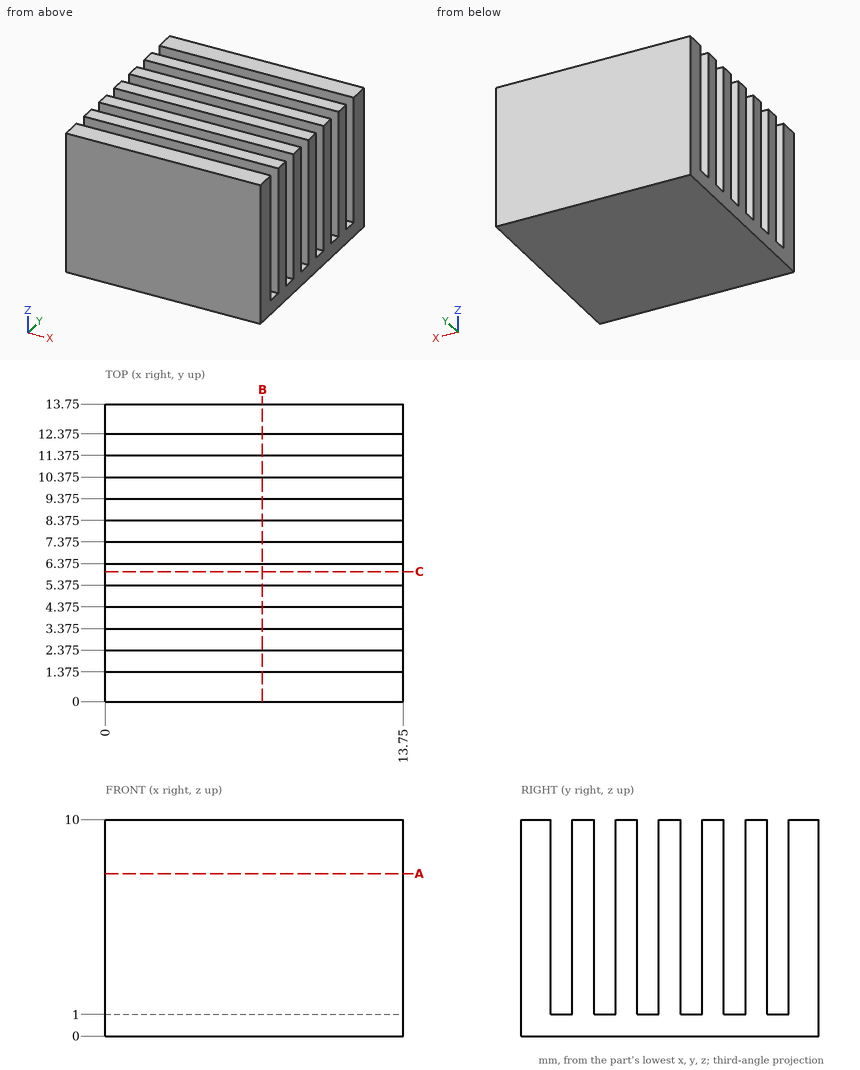
Geometry check sheet. Reference: drawing and pictorial views, mm from the part's lowest x, y, z. Round coordinates to 2 decimals unless told otherwise and drop trailing zeros. Loops run counter-clockwise (first coordinate to the right, second up) from the corner with the lowest first, then second, coordinate; pieces in that order, holes last. Notation, with made-up numbers: (87, 16.25) - (122, 16.25) arc R20 ccw to (122, 27.25) - close; hole circle Ø10 at (37, -5). An arc over 180 degrees is marked (long way). Answer in a Markdown table with one row per item. Add a question column.
Q1. Gauge pin test, flat ends, axial feed: pin 1 (1.1 mm diameter, centred on x = 9.5, y = 10, fed in from +Z); pin 2 (0.5 mm diameter, centred on x = 10, y = 6, fed in from +Z). Record the tip position at first contact, or that the pin passes through.
Q2. Section check A-A on z = 7.5. Enter the section's corners in (x, y) (3 decimals).
Q3. Section check B-B on x = 7.25. Enter the section's corners in (y, z) (3 decimals), plus the area to 3 significant figures.
Q4. Section check C-C on y = 6. Enter the section's corners in (x, z), plus the area to 4 significant figures.
Q5. Material ranges on line 1 (Z direction, x = 3, y = 7.5), recorded low to high.
Found:
| question | item | result |
|---|---|---|
| 1 | pin 1 | stops at z = 10 |
| 1 | pin 2 | stops at z = 1 |
| 2 | outline | (0, 0) - (13.75, 0) - (13.75, 1.375) - (0, 1.375) - close; (0, 2.375) - (13.75, 2.375) - (13.75, 3.375) - (0, 3.375) - close; (0, 4.375) - (13.75, 4.375) - (13.75, 5.375) - (0, 5.375) - close; (0, 6.375) - (13.75, 6.375) - (13.75, 7.375) - (0, 7.375) - close; (0, 8.375) - (13.75, 8.375) - (13.75, 9.375) - (0, 9.375) - close; (0, 10.375) - (13.75, 10.375) - (13.75, 11.375) - (0, 11.375) - close; (0, 12.375) - (13.75, 12.375) - (13.75, 13.75) - (0, 13.75) - close |
| 3 | outline | (0, 0) - (13.75, 0) - (13.75, 10) - (12.375, 10) - (12.375, 1) - (11.375, 1) - (11.375, 10) - (10.375, 10) - (10.375, 1) - (9.375, 1) - (9.375, 10) - (8.375, 10) - (8.375, 1) - (7.375, 1) - (7.375, 10) - (6.375, 10) - (6.375, 1) - (5.375, 1) - (5.375, 10) - (4.375, 10) - (4.375, 1) - (3.375, 1) - (3.375, 10) - (2.375, 10) - (2.375, 1) - (1.375, 1) - (1.375, 10) - (0, 10) - close |
| 3 | area | 83.5 mm² |
| 4 | outline | (0, 0) - (13.75, 0) - (13.75, 1) - (0, 1) - close |
| 4 | area | 13.75 mm² |
| 5 | line 1 | z = 0 to 1 |
